CAD build for the part. Positions are in the model's coordinates, mm. Face numbers are marked on the shaded views. Give positions to 0.01 mm unless a question says otherwise; leave off trailing zeros. Order: outer loops, then holes, each group sorted by start corner. A loop starts at its lowest first (then second) coordinate and runs counter-clockwise, first axis right, second up. Notation, with made-up numbers: M 40.25,-24.75 L 58.25,-24.75 A14 cw 58.25,-19.75 Z; hole C -40,84.5 d1. An arc over 180 degrees is marked long. Put each result on its own line as item: value. Start each with the question number.
1) Pin check, flat tips, straight feed: pin 1 (6 mm diameter, centred on y = -4, z = 14.5, fed in from -X); pin 2 (3 mm diameter, centred on x = 12.5, y = -3.5, fed in from -Z); pin 3 (1 mm diameter, centred on x = 7.5, y = -6.5, fed in from -Z). Stop position of each tip, or through.
2) Drill centre lines: line 1 (Y direction, x = -5.5, z = 30) (3 decimals); line 2 (Z direction, x = -20, y = -2); line 3 (Z direction, x = 0.5, y = -0.5). Where is each one in solid material? Low to high. Write a range as [from, to].
3) Cut at C-C (x = -8.5). Write the cut outline in (y, z) (3 decimals), and give its area (3 significant figures).
4) Cut at A-A (y = -4.5). Write the cut outline in (x, z), and give its area (3 significant figures).
5) Cut at B-B (z = 32). Write the cut outline in (x, y) (3 decimals), and give its area (3 significant figures).
6) Two-plate mould, pull along Y, no slides. Class the marked faces 1, 2 and 3: released by +Y, released by -Y, zero draft, split by the parting line, or undercut.
7) Cut at D-D (x = 29). Write the cut outline in (y, z) (3 decimals), and give its area (3 significant figures).
```python
from build123d import *

# Parameters (mm, degrees)
F0_W      = 203.2
F0_H      = 44.45
F1_DEPTH  = 3.175
F3_DEPTH  = 6.35
F5_DEPTH  = 25.4
F6_DEPTH  = 25.4
F8_DEPTH  = 12.7
F9_R      = 5.08
F10_DEPTH = 76.2
F12_DEPTH = 25.4


with BuildPart() as f1:
    # F0 (on Front) → F1 (new body, symmetric)
    with BuildSketch(Plane.XZ):
        with Locations((2.1883048997, 22.225)):
            Rectangle(F0_W, F0_H)
    extrude(amount=F1_DEPTH, both=True)

    # F2 (on face) → F3 (join, symmetric)
    with BuildSketch(Plane.XZ.offset(3.175)):
        Polygon((2.2116978689, -13.6960168671), (38.1093217669, 22.2483929692), (2.1649119306, 58.1460168671), (-33.7327119674, 22.2016070308), align=None)
    extrude(amount=F3_DEPTH, both=True)


with BuildPart() as f1_1:
    # F4: moved
    add(f1.part.moved(Location((-2.20971, 0, 0))))

    # F5 (cut): a face of the model
    f5_faces = [f1_1.faces().sort_by_distance(p)[0] for p in [
        (-62.9576531363, -3.175, 22.225592552),
    ]]
    extrude(f5_faces, amount=-F5_DEPTH, mode=Mode.SUBTRACT)

    # F6 (cut): a face of the model
    f6_faces = [f1_1.faces().sort_by_distance(p)[0] for p in [
        (62.9148429358, -3.175, 22.224407448),
    ]]
    extrude(f6_faces, amount=-F6_DEPTH, mode=Mode.SUBTRACT)

    # F7 (on face) → F8 (join)
    with BuildSketch(Plane.XZ.offset(9.525)):
        Polygon((35.8996117669, 58.1460168671), (-0.0447980694, 58.1460168671), (35.8996117669, 22.2483929692), align=None)
        Polygon((-35.9424219674, 22.2016070308), (-0.0447980694, 58.1460168671), (-35.9424219674, 58.1460168671), align=None)
    extrude(amount=-F8_DEPTH)

    # F9 (on face) → F10 (cut)
    with BuildSketch(Plane.YZ.offset(35.8996117669)):
        with Locations((-3.175, 30.1041658968)):
            Circle(F9_R)
    extrude(amount=-F10_DEPTH, mode=Mode.SUBTRACT)

    # F11 (on face) → F12 (cut)
    with BuildSketch(Plane.XZ.offset(9.525)):
        Polygon((35.8996117669, 58.1460168671), (-0.0447980694, 58.1460168671), (35.8996117669, 22.2483929692), align=None)
        Polygon((-35.9424219674, 58.1460168671), (-35.9424219674, 22.2016070308), (-0.0447980694, 58.1460168671), align=None)
    extrude(amount=-F12_DEPTH, mode=Mode.SUBTRACT)


solid = f1_1.part
```
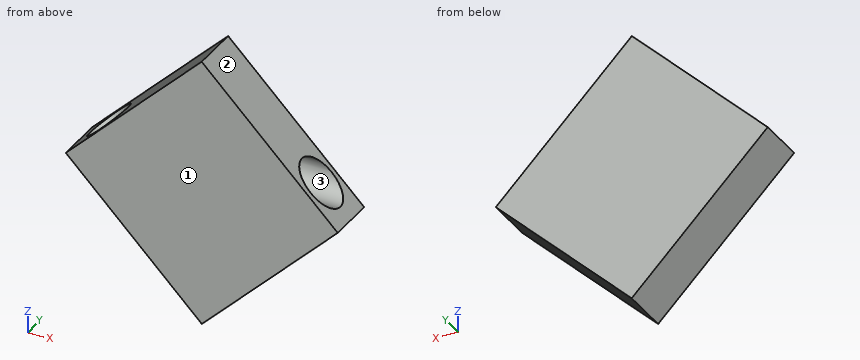
Solution:
1. pin 1: x = -31.23
1. pin 2: z = -2.68
1. pin 3: z = -6.69
2. line 1: [-9.525, -8.254], [1.904, 3.175]
2. line 2: [6.28, 25.16], [35.05, 38.16]
2. line 3: [-13.2, 25.79], [34.42, 57.6]
3. outline: M -9.525,-5.205 L 3.175,-5.205 L 3.175,49.68 L -9.525,49.68 Z; hole C -3.175,30.104 d10.16
3. area: 616 mm²
4. outline: M -35.94,22.2 L 0,-13.7 L 35.9,22.25 L 32.94,25.2 L -32.95,25.2 Z; M -23.15,35.01 L 23.12,35.01 L -0.04,58.15 Z
4. area: 2,030 mm²
5. outline: M -26.157,-9.525 L 26.135,-9.525 L 26.135,-7.888 L -26.157,-7.888 Z; M -26.157,1.538 L 26.135,1.538 L 26.135,3.175 L -26.157,3.175 Z
5. area: 171 mm²
6. face 1: released by -Y
6. face 2: zero draft
6. face 3: undercut
7. outline: M -9.525,15.34 L 3.175,15.34 L 3.175,29.139 L 1.812,29.139 A5.08 cw -8.162,29.139 L -9.525,29.139 Z
7. area: 144 mm²
